```python
from build123d import *

# Parameters (mm, degrees)
F12_DEPTH = 1.3094010768
F13_R     = 4
F14_R     = 2
F15_COUNT = 3


with BuildPart() as f12:
    # F11 (on 3pt) → F12 (new body)
    with BuildSketch(Plane(origin=(12.4766063631, -0.6238303182, 7.2033720423), x_dir=(0.0374648931, 0.9990638163, 0.0216303661), z_dir=(0.8652146449, -0.0432607322, 0.4995319082))):
        Polygon((-199.5629973065, -10), (0.6244148852, -25), (0.6244148852, 25), (-199.5629973065, 10), align=None)
        Polygon((-195.5629973065, -6.2885059162), (-195.5629973065, 6.2885059162), (-187.6440477443, 6.881871114), (-132.2063387469, 11.0358067979), (-128.2063387469, 11.3355259428), (-120.5510228532, 11.9091371262), (-66.0701318871, 15.9913786395), (-62.0701318871, 16.2910977844), (-54.4132921405, 16.8648231497), (-3.3755851148, 20.6890676264), (-3.3755851148, -20.6890676264), (-12.7686794815, -19.9852450736), (-62.0701318871, -16.2910977844), (-66.0701318871, -15.9913786395), (-76.3495546331, -15.2211436906), (-128.2063387469, -11.3355259428), (-132.2063387469, -11.0358067979), (-144.9052103128, -10.0842830662), align=None, mode=Mode.SUBTRACT)
        Polygon((-187.6440477443, 6.881871114), (-195.5629973065, 6.2885059162), (-144.9052103128, -10.0842830662), (-132.2063387469, -11.0358067979), align=None)
        Polygon((-128.2063387469, 11.3355259428), (-132.2063387469, 11.0358067979), (-132.2063387469, -11.0358067979), (-128.2063387469, -11.3355259428), align=None)
        Polygon((-120.5510228532, 11.9091371262), (-128.2063387469, 11.3355259428), (-76.3495546331, -15.2211436906), (-66.0701318871, -15.9913786395), align=None)
        Polygon((-62.0701318871, 16.2910977844), (-66.0701318871, 15.9913786395), (-66.0701318871, -15.9913786395), (-62.0701318871, -16.2910977844), align=None)
        Polygon((-54.4132921405, 16.8648231497), (-62.0701318871, 16.2910977844), (-12.7686794815, -19.9852450736), (-3.3755851148, -20.6890676264), align=None)
    extrude(amount=-F12_DEPTH)

    # F13
    f13_edges = [f12.edges().sort_by_distance(p)[0] for p in [
        (7.727656, -195.975422, -2.799777),
        (12.474957, -132.678077, -5.540632),
        (12.774676, -128.681822, -5.713675),
        (22.128218, -3.967932, -11.113945),
        (1.43915, -3.967932, 24.720571),
        (1.43915, -66.603786, 19.296147),
        (1.43915, -62.60753, 19.642233),
        (1.43915, -195.975422, 8.092235),
        (1.43915, -132.678077, 13.573946),
        (1.43915, -128.681822, 13.920032),
        (17.430529, -66.603786, -8.401733),
        (17.730248, -62.60753, -8.574776),
    ]]
    fillet(f13_edges, radius=F13_R)

    # F14
    f14_edges = [f12.edges().sort_by_distance(p)[0] for p in [
        (1.43915, -121.033672, 14.582381),
        (1.43915, -188.063886, 8.777394),
        (11.523433, -145.36506, -4.99127),
        (16.660294, -76.873585, -7.957038),
        (1.43915, -54.957859, 20.304714),
        (21.424395, -13.352233, -10.707593),
    ]]
    fillet(f14_edges, radius=F14_R)


with BuildPart() as f15_1:
    # F15: instance of F12
    add(f12.part.rotate(Axis((0, -100, 0), (0, -1, 0)), 1 * 360 / F15_COUNT))


with BuildPart() as f15_2:
    # F15: instance of F12
    add(f12.part.rotate(Axis((0, -100, 0), (0, -1, 0)), 2 * 360 / F15_COUNT))


with BuildPart() as f17_1:
    # F17: instance of F12
    add(f12.part.mirror(Plane.YZ))


with BuildPart() as f18_tool:
    # F6 (on Front) → F18 section 0
    with BuildSketch(Plane.XZ):
        Polygon((-25, -14.4337567297), (25, -14.4337567297), (0, 28.8675134595), align=None)
    # F8 (on offset) → F18 section 1
    with BuildSketch(Plane.XZ.offset(200)):
        Polygon((10, -5.7735026919), (0, 11.5470053838), (-10, -5.7735026919), align=None)
    loft()


with BuildPart() as f12_1:
    add(f12.part)

    # F18: intersect by f18_tool
    add(f18_tool.part, mode=Mode.INTERSECT)


with BuildPart() as f15_2_1:
    add(f15_2.part)

    # F18: intersect by f18_tool
    add(f18_tool.part, mode=Mode.INTERSECT)


with BuildPart() as f17_1_1:
    add(f17_1.part)

    # F18: intersect by f18_tool
    add(f18_tool.part, mode=Mode.INTERSECT)


with BuildPart() as f12_2:
    add(f12_1.part)

    # F19: union F15_2, F17_1
    add(f15_2_1.part)
    add(f17_1_1.part)


solid = f12_2.part
```
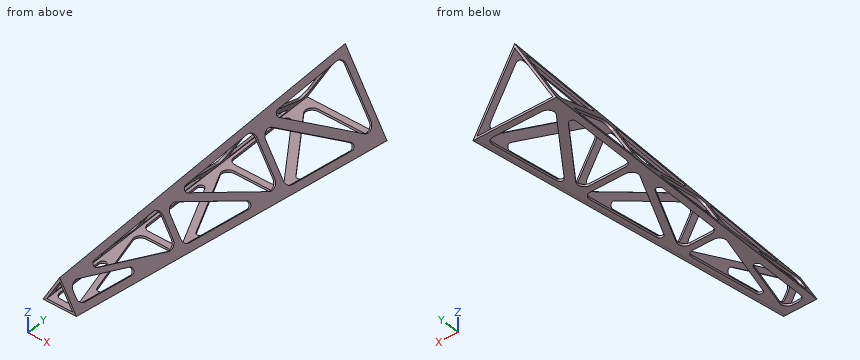
Geometry: final body of the model. Coordinates: model frame, mm. Coordinates: 2 decimals unless noted, no trailing zeros. Answer as CSV lines item,"result". Start each with the question number.
Q1. Line query: line 1 (Z direction, x = 19, y = -48); line 2 (Z direction, x = -14.5, y = -107); line 3 (Y direction, x = -16.5, z = -1). Output: solid intervals per line, ascending. Write a range as from..to.
Q2. Pin query (flat end, axial travel): P1, Ø2, axis at y = -47, z = 17, coming from the +X side; P2, Ø8, axis at x = 13, y = -173, coming from the -Z side; P3, Ø1, axis at x = 8.5, z = 3.5, coming from the -Y side; P4, Ø1, axis at x = 1.5, y = -67, coming from the +Z side. Return the tip coordinate at first contact, or that it passes through.
Q3. Cut plane A-A on y = -23.5. Count the separate pieces of the cut face and the enclosed holes in it, then the cut area to 3 significant figures.
Findings below:
1,line 1,"z = -12.36..-11.04, -10.82..-9.11"
1,line 2,"z = -9.8..-8.49, -8.13..-6.6"
1,line 3,"y = -3.98..0"
2,P1,"passes through"
2,P2,"stops at z = -7.11"
2,P3,"stops at y = -132.71"
2,P4,"stops at z = 21.33"
3,separate pieces,"6"
3,enclosed holes,"0"
3,area,"47.0 mm2"
